```python
from build123d import *

# Parameters (mm, degrees)
SKETCH1_R           = 7.5
SKETCH1_R_2         = 1.75
BOSS_EXTRUDE1_DEPTH = 28
CUT_EXTRUDE1_DEPTH  = 30.941609843
CIRPATTERN1_COUNT   = 5


with BuildPart() as part:
    # Sketch1 → Boss-Extrude1 (new body)
    with BuildSketch(Plane.XY):
        Circle(SKETCH1_R)
        Circle(SKETCH1_R_2, mode=Mode.SUBTRACT)
    extrude(amount=BOSS_EXTRUDE1_DEPTH)

    # Sketch2 → Cut-Extrude1 (cut, through all)
    with BuildSketch(Plane.XY):
        Polygon((0, 3.429306859), (-1.35645876, 4.852854397), (-4.219139018, 6.200714954), (0, 11.25164702), (4.219139018, 6.200714954), (1.35645876, 4.852854397), align=None)
    cut_extrude1 = extrude(amount=CUT_EXTRUDE1_DEPTH, mode=Mode.SUBTRACT)

    # CirPattern1: Cut-Extrude1 ×5 about axis
    cirpattern1_axis = Axis((0, 0, 0), (0, 0, 1))
    for i in range(1, CIRPATTERN1_COUNT):
        add(cut_extrude1.rotate(cirpattern1_axis, i * 360 / CIRPATTERN1_COUNT), mode=Mode.SUBTRACT)


solid = part.part
```
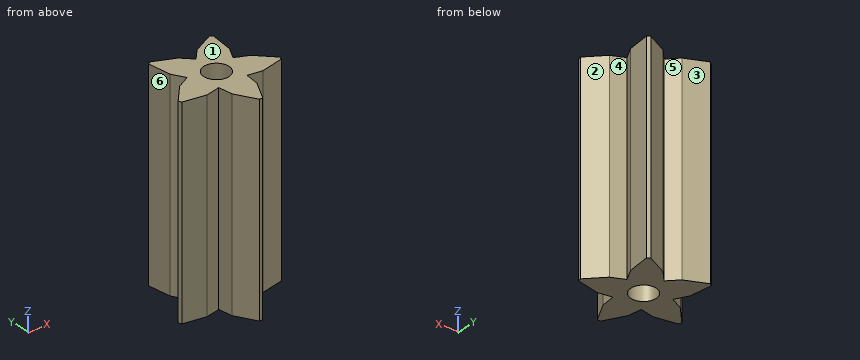
Source: CAD feature listing. Evaluate the final solid. Frame: model axes, mm. Face numbers are marked on the shaded views. A direction names the side the tool comes from. Give positions to 0.01 mm unless a question says otherwise; leave off trailing zeros. Loops run counter-clockwise (first coordinate to the right, second up) from the corner with the lowest first, then second, coordinate; pieces in that order, holes last. Notation, with made-up numbers: (-34.75, 72) - (-25.75, 72) arc R16 ccw to (-25.75, 99) - close; hole circle Ø5 at (31, 37.5). An arc over 180 degrees is marked (long way). Use CSV: the item, a comma, the result in double quotes. Start each with the question number.
1. Section C-C (y = -5.5). Output: boundary loops of the cut face in (x, z).
2. Ray query, L1, parallel to X at y = 3, z = 5; L2, parallel to Y at x = -0.75, z = 14.5; L3, parallel to Y at x = -1, z = 4.75. Return the intervals inside material, ascending.
3. Pin query (flat end, axial travel): pin 1 (1 mm diameter, centred on y = 1.5, z = 22, fed in from -X); pin 2 (1 mm diameter, centred on y = -4.5, z = 10.5, fed in from -X); pin 3 (4 mm diameter, centred on x = -4.5, z = 6, fed in from +Y). Return the tip coordinate at first contact, or that it passes through.
4. Reachability of the marked faces 4, 5 and 6 from +Z, -Z, +X, -X, +Y, -Y: full face, straight path, thin tool, end or side. Return the list, or none.
5. Draft query along X for the marked faces 1, 2 and 3. Return one class per face: +X half, -X half, draft (parallel to the pull), parting line (faces both ways), or undercut.
6. Section D-D (y = 2.25). Output: boundary loops of the cut face in (x, z), then the cut area to 3 significant figures.
7. Section B-B (y = -0.75). Output: boundary loops of the cut face in (x, z).
8. Section A-A (z = 2.25). Output: boundary loops of the cut face in (x, y), then the cut area to 3 significant figures.
Response:
1,outline,"(-1.33, 0) - (1.33, 0) - (1.33, 28) - (-1.33, 28) - close"
2,L1,"-4.22 to 4.22"
2,L2,"-6.55 to -1.58, 1.58 to 4.22"
2,L3,"-6.1 to -1.44, 1.44 to 4.48"
3,pin 1,"x = -3.77"
3,pin 2,"x = -1.85"
3,pin 3,"y = 6.2"
4,face 4,"+Z, -Z, +X"
4,face 5,"+Z, -Z, +Y"
4,face 6,"+Z, -Z, -X"
5,face 1,"draft"
5,face 2,"+X half"
5,face 3,"undercut"
6,outline,"(-3.9, 0) - (3.9, 0) - (3.9, 28) - (-3.9, 28) - close"
6,area,"219 mm²"
7,outline,"(-5.94, 0) - (-1.58, 0) - (-1.58, 28) - (-5.94, 28) - close; (1.58, 0) - (5.94, 0) - (5.94, 28) - (1.58, 28) - close"
8,outline,"(-7.2, -2.1) arc R7.5 ccw to (-7.06, -2.54) - (-3.95, -3.13) - (-2.02, -2.77) - (-1.76, -4.72) - (-0.23, -7.5) arc R7.5 ccw to (0.23, -7.5) - (1.76, -4.72) - (2.02, -2.77) - (3.95, -3.13) - (7.06, -2.54) arc R7.5 ccw to (7.2, -2.1) - (5.03, 0.21) - (3.26, 1.06) - (4.2, 2.79) - (4.59, 5.93) arc R7.5 ccw to (4.22, 6.2) - (1.36, 4.85) - (0, 3.43) - (-1.36, 4.85) - (-4.22, 6.2) arc R7.5 ccw to (-4.59, 5.93) - (-4.2, 2.79) - (-3.26, 1.06) - (-5.03, 0.21) - close; hole circle Ø3.5 at (0, 0)"
8,area,"82.6 mm²"
